```python
from build123d import *

# Parameters (mm, degrees)
F1_DEPTH = 30
F2_R     = 2
F3_DEPTH = 25
F4_R     = 2
F5_DEPTH = 10
F6_R     = 3
F7_R     = 1.5


with BuildPart() as f1:
    # F0 (on Front) → F1 (new body, symmetric)
    with BuildSketch(Plane.XZ):
        Polygon((92.5, 80), (0, 80), (-92.5, 80), (-92.5, 0), (-67.5, 0), (-67.5, 1.5), (-91, 1.5), (-91, 78.5), (0, 78.5), (91, 78.5), (91, 1.5), (67.5, 1.5), (67.5, 0), (92.5, 0), align=None)
    extrude(amount=F1_DEPTH, both=True)

    # F2 (on face) → F3 (cut)
    with BuildSketch(Plane.XY.offset(80)):
        with Locations((-66.5, 20)):
            Circle(F2_R)
        with Locations((-66.5, -20)):
            Circle(F2_R)
        with Locations((66.5, 20)):
            Circle(F2_R)
        with Locations((66.5, -20)):
            Circle(F2_R)
    extrude(amount=-F3_DEPTH, mode=Mode.SUBTRACT)

    # F4 (on face) → F5 (cut)
    with BuildSketch(Plane(origin=(0, 0, 0), x_dir=(1, 0, 0), z_dir=(0, 0, -1))):
        with Locations((-80, 20)):
            Circle(F4_R)
        with Locations((-80, -20)):
            Circle(F4_R)
        with Locations((80, -20)):
            Circle(F4_R)
        with Locations((80, 20)):
            Circle(F4_R)
    extrude(amount=-F5_DEPTH, mode=Mode.SUBTRACT)

    # F6
    f6_edges = [f1.edges().sort_by_distance(p)[0] for p in [
        (-92.5, 0, 80),
        (-92.5, 0, 0),
        (92.5, 0, 80),
        (92.5, 0, 0),
    ]]
    fillet(f6_edges, radius=F6_R)

    # F7
    f7_edges = [f1.edges().sort_by_distance(p)[0] for p in [
        (-91, 0, 78.5),
        (91, 0, 78.5),
        (-91, 0, 1.5),
        (91, 0, 1.5),
    ]]
    fillet(f7_edges, radius=F7_R)


solid = f1.part
```
Check sheet for the modelled part. Datum: model origin and axes. Units: mm. A direction names the side the tool comes from. Coordinates: 2 decimals unless noted, no trailing zeros. Write each loop counter-clockwise with the first axis right and the second up, starting at its lowest first coordinate (ties: lowest second). Pieces come first, ordered by that corner, then holes. Notation, with made-up numbers: M 75,-39.75 L 80,-39.75 A12 cw 80,-22.75 Z; hole C 44,66 d6. An arc over 180 degrees is marked long. Write item = value, one per line. Start each with the question number.
1. Sectioned sample at A-A (x = 80). Record the cut outline in (y, z).
2. Sectioned sample at C-C (y = -6). Record the cut outline in (x, z), then the cut area to 3 significant figures.
3. Sectioned sample at D-D (y = 20). State how many separate pieces and enclosed holes the cut face has, then the cut area to 3 significant figures.
4. Sectioned sample at B-B (z = 60). Record the cut outline in (x, y), then the cut area to 3 significant figures.
5. Thickness scan on probe 1 along X at (y, z) = (20, 0.4); probe 2 along X at (y, z) = (6, 25.5); probe 3 along Z at (x, y) = (82.5, 1). Record the ranges inside material, lowest first.
6. Go/stop test with flat-tipped pins: pin 1 (2 mm diameter, centred on x = -26, y = -7.5, fed in from -Z); pin 2 (3 mm diameter, centred on x = 66.5, y = -20, fed in from +Z); pin 3 (1.2 mm diameter, centred on y = -8.5, z = 1, fed in from -X). Record where each tip stops, or that it passes through.
7. Tool access check on faces 5 (the flat face through (79, 0, 1.5)), 6 (the flat face through (0, -30, 79)), 7 (the cylindrical face through (66.24, 21.983, 79.26)), 8 (the cylindrical face through (81.908, -20.601, 0.74)), 9 (the flat face through (92.5, 0, 39)). Record the directions out of +Z, -Z, +X, -X, +Y, -Y that give a thin tool (end or side, any length) a straight path to the whole face; none if there is none.
8. Mould release check, pull along Z, two halves, no side actions. Record for faces 1 (the flat face through (-1, 0, 78.5)), 2 (the flat face through (91, 0, 41)), 3 (the flat face through (-92.5, 0, 41)), 4 (the flat face through (-79, 0, 0)): pulls with the +Z half, pulls with the -Z half, needs draft (parallel to the pull), parting line crosses it, or undercut.
The answers:
q1.outline = M -30,0 L -22,0 L -22,1.5 L -30,1.5 Z; M -30,78.5 L 30,78.5 L 30,80 L -30,80 Z; M -18,0 L 18,0 L 18,1.5 L -18,1.5 Z; M 22,0 L 30,0 L 30,1.5 L 22,1.5 Z
q2.outline = M -92.5,3 A3 ccw -89.5,0 L -67.5,0 L -67.5,1.5 L -89.5,1.5 A1.5 cw -91,3 L -91,77 A1.5 cw -89.5,78.5 L 89.5,78.5 A1.5 cw 91,77 L 91,3 A1.5 cw 89.5,1.5 L 67.5,1.5 L 67.5,0 L 89.5,0 A3 ccw 92.5,3 L 92.5,77 A3 ccw 89.5,80 L -89.5,80 A3 ccw -92.5,77 Z
q2.area = 578 mm²
q3.separate_pieces = 5
q3.enclosed_holes = 0
q3.area = 554 mm²
q4.outline = M -92.5,-30 L -91,-30 L -91,30 L -92.5,30 Z; M 91,-30 L 92.5,-30 L 92.5,30 L 91,30 Z
q4.area = 180 mm²
q5.probe_1 = -91 to -82, -78 to -67.5, 67.5 to 78, 82 to 91
q5.probe_2 = -92.5 to -91, 91 to 92.5
q5.probe_3 = 0 to 1.5, 78.5 to 80
q6.pin_1 = 78.5
q6.pin_2 = 1.5
q6.pin_3 = -92.15
q7.face_5 = +Y, -Y
q7.face_6 = +Z, -Z, +X, -X, -Y
q7.face_7 = +Z
q7.face_8 = -Z
q7.face_9 = +Z, -Z, +X, +Y, -Y
q8.face_1 = undercut
q8.face_2 = undercut
q8.face_3 = needs draft
q8.face_4 = pulls with the -Z half
